Input: part model. Units: mm. Frame: model coordinates. A direction names the side the tool comes from. Give positions to 0.01 mm unless a question says otherwise; leave off trailing zeros. Loops run counter-clockwise (first coordinate to the right, second up) from the corner with the lowest first, then second, coordinate; pieces in that order, holes last. Notation, with made-up numbers: (-25.5, 48) -> (27.5, 48) arc R23 ccw to (27.5, 71) -> close; hole circle Ø9 at (43.25, 76.5). An arc over 180 degrees is marked (long way). Use CSV: the item, a comma, the result in double quotes.
```python
from build123d import *

# Parameters (mm, degrees)
F0_R      = 30.95625
F0_R_2    = 22.225
F1_DEPTH  = 92.075
F2_R      = 40.48125
F2_R_2    = 30.95625
F3_DEPTH  = 6.35
F4_R      = 40.48125
F4_R_2    = 30.95625
F5_DEPTH  = 6.35
F13_R     = 7.9375
F15_R     = 2.54
F16_DEPTH = 17.4625
F17_R     = 2.54
F18_DEPTH = 22.2377
F19_R     = 4.7625
F20_DEPTH = 16.002


with BuildPart() as f1:
    # F0 (on Top) → F1 (new body)
    with BuildSketch(Plane.XY):
        Circle(F0_R)
        Circle(F0_R_2, mode=Mode.SUBTRACT)
    extrude(amount=F1_DEPTH)

    # F2 (on face) → F3 (join)
    with BuildSketch(Plane.XY.offset(92.075)):
        Circle(F2_R)
        Circle(F2_R_2, mode=Mode.SUBTRACT)
    extrude(amount=-F3_DEPTH)

    # F4 (on face) → F5 (join)
    with BuildSketch(Plane(origin=(0, 0, 0), x_dir=(1, 0, 0), z_dir=(0, 0, -1))):
        Circle(F4_R)
        Circle(F4_R_2, mode=Mode.SUBTRACT)
    extrude(amount=-F5_DEPTH)

    # F7 (on offset) → F8 (join, up to the next surface of F1)
    with BuildSketch(Plane.XZ.offset(58.7375)):
        Polygon((-8.73125, 73.025), (0, 73.025), (8.73125, 73.025), (8.73125, 85.725), (-8.73125, 85.725), align=None)
    extrude(until=Until.NEXT, dir=(0, 1, 0))

    # F10 (on offset) → F11 (join, up to the next surface of F1)
    with BuildSketch(Plane.XZ.offset(52.3875)):
        Polygon((11.1125, 15.875), (0, 15.875), (-11.1252, 15.875), (-11.1252, 6.35), (11.1125, 6.35), align=None)
    extrude(until=Until.NEXT, dir=(0, 1, 0))

    # F13 (on offset) → F14 (join, up to the next surface of F1)
    with BuildSketch(Plane.YZ.offset(-37.30625)):
        with Locations((0, 46.0375)):
            Circle(F13_R)
    extrude(until=Until.NEXT)

    # F15 (on face) → F16 (cut, through all)
    with BuildSketch(Plane(origin=(-8.73125, 0, 0), x_dir=(0, -1, 0), z_dir=(-1, 0, 0))):
        with BuildLine():
            ThreePointArc((52.3874999998, 85.725), (56.8776280605, 83.8651280606), (58.7375, 79.375))
            Line((58.7375, 79.375), (58.7375, 85.725))
            Line((58.7374999992, 85.725), (52.3874999994, 85.725))
        make_face()
        with BuildLine():
            ThreePointArc((58.7375, 79.375), (56.8776280605, 74.8848719394), (52.3874999998, 73.025))
            Line((52.3874999994, 73.025), (58.7374999992, 73.025))
            Line((58.7375, 73.025), (58.7375, 79.375))
        make_face()
        with Locations((52.3875, 79.375)):
            Circle(F15_R)
    extrude(amount=-F16_DEPTH, mode=Mode.SUBTRACT)

    # F17 (on face) → F18 (cut, through all)
    with BuildSketch(Plane(origin=(-11.1252, 0, 0), x_dir=(0, -1, 0), z_dir=(-1, 0, 0))):
        with BuildLine():
            ThreePointArc((47.6249999998, 15.875), (50.9925960453, 14.4800960455), (52.3875, 11.1125))
            Line((52.3875, 11.1125), (52.3875, 15.875))
            Line((52.3874999992, 15.875), (47.6249999994, 15.875))
        make_face()
        with BuildLine():
            ThreePointArc((52.3875, 11.1125), (50.9925960453, 7.7449039545), (47.6249999998, 6.35))
            Line((47.6249999994, 6.35), (52.3874999992, 6.35))
            Line((52.3875, 6.35), (52.3875, 11.1125))
        make_face()
        with Locations((47.625, 11.1125)):
            Circle(F17_R)
    extrude(amount=-F18_DEPTH, mode=Mode.SUBTRACT)

    # F19 (on face) → F20 (cut)
    with BuildSketch(Plane(origin=(-37.30625, 0, 0), x_dir=(0, -1, 0), z_dir=(-1, 0, 0))):
        with Locations((0, 46.0375)):
            Circle(F19_R)
    extrude(amount=-F20_DEPTH, mode=Mode.SUBTRACT)


solid = f1.part
```
1) Section query A-A (x = 0). Give the number of separate pieces and of enclosed holes in the cut face, then the cut area to 3 significant figures.
From the geometry:
separate pieces,"2"
enclosed holes,"2"
area,"2,340 mm^2"
2) Mould query, pull axis Z, two halves, no side actions, for faces 5 (the cylindrical face through (20.53, -8.51, 45.39)), 6 (the flat face through (0, -46, 85.725)), 7 (the cylindrical face through (-33.665, 3.663, 38.996)). Classes: pulls with the +Z half, pulls with the -Z half, needs draft (parallel to the pull), parting line crosses it, or undercut.
From the geometry:
face 5,"needs draft"
face 6,"pulls with the +Z half"
face 7,"undercut"
3) Reachability of faces 1 (the cylindrical face through (-29.617, 1.032, 41.388)), 2 (the flat face through (-15.2, 27.3, 85.725)), 3 (the flat face through (-11.125, -38, 11)), 4 (the flat face through (8.731, -44, 79)) from +Z, -Z, +X, -X, +Y, -Y: full face, straight path, thin tool, end or side. Return the list, or none.
From the geometry:
face 1,"-X"
face 2,"none"
face 3,"-X, -Y"
face 4,"+X, -Y"
4) Ray query, line 1 (Y direction, x = 0, z = 26) (3 decimals); line 2 (Y direction, x = 8, z = 79); line 3 (Z direction, x = 27.5, y = -24) (3 decimals). Return the intervals inside material, ascending.
From the geometry:
line 1,"y = -30.956 to -22.225, 22.225 to 30.956"
line 2,"y = -58.73 to -54.9, -49.88 to -20.74, 20.74 to 29.9"
line 3,"z = 0 to 6.35, 85.725 to 92.075"
5) Section query B-B (y = 0). Return loops of the section in (x, z) (3 decimals), then the cut area to 3 significant figures.
From the geometry:
outline,"(-40.481, 0) -> (-22.225, 0) -> (-22.225, 41.275) -> (-37.306, 41.275) -> (-37.306, 38.1) -> (-30.956, 38.1) -> (-30.956, 6.35) -> (-40.481, 6.35) -> close; (-40.481, 85.725) -> (-30.956, 85.725) -> (-30.956, 53.975) -> (-37.306, 53.975) -> (-37.306, 50.8) -> (-22.225, 50.8) -> (-22.225, 92.075) -> (-40.481, 92.075) -> close; (22.225, 0) -> (40.481, 0) -> (40.481, 6.35) -> (30.956, 6.35) -> (30.956, 85.725) -> (40.481, 85.725) -> (40.481, 92.075) -> (22.225, 92.075) -> close"
area,"1,810 mm^2"
6) Contact query for flat-ended pins moving along their axis: pin 1 (4.5 mm diameter, centred on x = -2, y = -43, fed in from -Z); pin 2 (12.5 mm diameter, centred on y = 0, z = 46.04, fed in from -X); pin 3 (2 mm diameter, centred on x = 2, z = 20, fed in from -Y); pin 4 (4.5 mm diameter, centred on y = -52.39, z = 79.38, fed in from +X). Output: stop coordinate, or through.
From the geometry:
pin 1,"stops at z = 6.35"
pin 2,"stops at x = -37.31"
pin 3,"stops at y = -30.94"
pin 4,"passes through"
